from build123d import *

# Parameters (mm, degrees)
ESQUISSE1_W                  = 90
ESQUISSE1_H                  = 240
BOSS_EXTRU_1_DEPTH           = 10
ENL_V_MAT_EXTRU_1_DEPTH      = 257.515106768
ENL_V_MAT_EXTRU_1_DEPTH_BACK = 257.515106768
ESQUISSE2_R                  = 1
ESQUISSE2_R_2                = 6


with BuildPart() as part:
    # Esquisse1 → Boss.-Extru.1 (new body)
    with BuildSketch(Plane.XY):
        with Locations((45, 120)):
            Rectangle(ESQUISSE1_W, ESQUISSE1_H)
    extrude(amount=BOSS_EXTRU_1_DEPTH)

    # Esquisse2 → Enlèv. mat.-Extru.1 (cut, two sides: drawn at the far end of the back side and taken through both)
    with BuildSketch(Plane.XY.offset(10).offset(-ENL_V_MAT_EXTRU_1_DEPTH_BACK)):
        with Locations((45, 54)):
            Circle(ESQUISSE2_R)
        with Locations((45, 38)):
            Circle(ESQUISSE2_R)
        with Locations((21, 9.5)):
            Circle(ESQUISSE2_R)
        with Locations(Location((69, 9.5, 0), (0, 0, 180))):
            Circle(ESQUISSE2_R)
        with Locations((45, 192)):
            Circle(ESQUISSE2_R_2)
        with Locations((45, 182)):
            Circle(ESQUISSE2_R)
        with Locations(Location((45, 202, 0), (0, 0, 180))):
            Circle(ESQUISSE2_R)
    extrude(amount=ENL_V_MAT_EXTRU_1_DEPTH + ENL_V_MAT_EXTRU_1_DEPTH_BACK, mode=Mode.SUBTRACT)


solid = part.part
Geometry: final body of the model. Coordinates: model frame, mm. Coordinates: 2 decimals unless noted, no trailing zeros. Loops run counter-clockwise (first coordinate to the right, second up) from the corner with the lowest first, then second, coordinate; pieces in that order, holes last. Notation, with made-up numbers: M 1.5,53 L 43.5,53 A26 ccw 43.5,69 Z; hole C 2.25,-1 d7. An arc over 180 degrees is marked long. One line per item, written item: value. Start each with the question number.
1) Draft query along X for faces 1 (the flat face through (0, 118, 5)), 2 (the flat face through (44, 122, 10)), 3 (the cylindrical face through (43.699, 186.143, 4.93)). Return one class per face: released by +X, released by -X, zero draft, split by the parting line, or undercut.
2) Material intervals for L1, parallel to Y at x = 45, z = 3; L2, parallel to X at y = 38, z = 5.25; L3, parallel to X at y = 192, z = 2.75, sorted ascending. Write a range as from..to.
3) Pin query (flat end, axial travel): P1, Ø1.8, axis at x = 45, y = 54, coming from the +Z side; P2, Ø1, axis at x = 41.5, z = 1.5, coming from the -Y side. Return the tip coordinate at first contact, or that it passes through.
4) Cut plane A-A (y = 192). Return loops of the section in (x, z), then the cut area to 3 significant figures.
Evaluation:
1. face 1: released by -X
1. face 2: zero draft
1. face 3: undercut
2. L1: 0..37, 39..53, 55..181, 183..186, 198..201, 203..240
2. L2: 0..44, 46..90
2. L3: 0..39, 51..90
3. P1: through
3. P2: y = 0
4. outline: M 0,0 L 39,0 L 39,10 L 0,10 Z; M 51,0 L 90,0 L 90,10 L 51,10 Z
4. area: 780 mm^2
